```python
from build123d import *

# Parameters (mm, degrees)
F1_DEPTH = 6.35
F3_D     = 1.524
F4_R     = 0.381


with BuildPart() as f1:
    # F0 (on Front) → F1 (new body)
    with BuildSketch(Plane.XZ):
        with BuildLine():
            Line((0, -7.4092204591), (0, 0))
            Line((0, 0), (-2.54, 0))
            Line((-2.54, 0), (-2.54, -4.318))
            ThreePointArc((-2.54, -4.318), (-2.9863692655, -5.3956307345), (-4.064, -5.842))
            Line((-4.064, -5.842), (-9.398, -5.842))
            Line((-9.398, -5.842), (-11.068511021, -7.3997767286))
            ThreePointArc((-11.068511021, -7.3997767286), (-5.53701683, -10.6408992323), (0, -7.4092204591))
        make_face()
    extrude(amount=F1_DEPTH)

    # F3 (through all)
    with Locations(Plane.YZ):
        with Locations((-3.175, -1.7639952663)):
            Hole(F3_D / 2)

    # F4
    f4_edges = [f1.edges().sort_by_distance(p)[0] for p in [
        (-2.54, -3.175, 0),
        (0, -3.175, 0),
        (-1.27, -6.35, 0),
        (-1.27, 0, 0),
        (0, -6.35, -3.70461),
        (-2.54, -6.35, -2.159),
        (-2.986369, -6.35, -5.395631),
        (-6.731, -6.35, -5.842),
        (-10.233256, -6.35, -6.620888),
        (-5.537017, -6.35, -10.640899),
        (0, -3.175, -7.40922),
        (-9.398, -3.175, -5.842),
        (-2.54, 0, -2.159),
        (-2.986369, 0, -5.395631),
        (-6.731, 0, -5.842),
        (-10.233256, 0, -6.620888),
        (-5.537017, 0, -10.640899),
        (0, 0, -3.70461),
        (-11.068511, -3.175, -7.399777),
        (0, -3.937, -1.763995),
        (-2.54, -3.937, -1.763995),
    ]]
    fillet(f4_edges, radius=F4_R)


solid = f1.part
```
Design review of the part built by this model. Coordinates are the model's own, in mm. A direction names the side the tool comes from. Round coordinates to 2 decimals unless told otherwise and drop trailing zeros. Order: outer loops, then holes, each group sorted by start corner. A loop starts at its lowest first (then second) coordinate and runs counter-clockwise, first axis right, second up. Notation, with made-up numbers: (-19.5, 21) - (29.5, 21) arc R10 cw to (29.5, 39) - close; hole circle Ø9 at (33.5, 27). An arc over 180 degrees is marked (long way). One line per question, with ' | ' between items.
Item 1: Draft analysis for pull direction Y (two halves, no side actions). For faces 3 (the face through (-10.11, -6.24, -6.66)), 4 (the face through (-1.28, -3.58, -1.12)), 5 (the face through (-10.11, -0.11, -6.66)), 6 (the face through (-5.52, -3.14, -10.64)), state which applies: +Y half, -Y half, draft (parallel to the pull), parting line (faces both ways), or undercut.
Checks:
face 3: -Y half | face 4: undercut | face 5: +Y half | face 6: draft
Item 2: For P1, Ø2, axis at y = -4, z = -3, coming from the -X side, flat-tipped, find the tip position at first contact; note if it passes through.
Checks:
P1: x = -2.54
Item 3: Wall thickness on line 1 (X direction, y = -1, z = -0.75); line 2 (X direction, y = -3.5, z = -7.5); line 3 (Z direction, x = -2, y = -2.5): over which ranges is each line inside the solid? List them lowest first. Write a range as [from, to].
Checks:
line 1: [-2.54, 0] | line 2: [-10.96, -0.05] | line 3: [-9.57, -2.12], [-1.41, 0]
Item 4: Machinability: for faces 1 (the face through (-4, 0, -7)), 2 (the face through (-7, -3, -5.842)), which of the approach directions +Z, -Z, +X, -X, +Y, -Y give a long, thin tool a straight path to every point of the face, cutting with its end or side? Answer none if there is none.
Checks:
face 1: +Z, -Z, +X, -X, +Y | face 2: +Z, -X, +Y, -Y
Item 5: Take a section at A-A, the plane y = -1.5. Write out the cut boundary in (x, z).
Checks:
outline: (-10.91, -7.67) arc R6.35 ccw to (-0.05, -7.5) arc R0.38 ccw to (0, -7.31) - (0, -0.38) arc R0.38 ccw to (-0.38, 0) - (-2.16, 0) arc R0.38 ccw to (-2.54, -0.38) - (-2.54, -4.32) arc R1.52 cw to (-4.06, -5.84) - (-9.25, -5.84) arc R0.38 ccw to (-9.51, -5.94) - (-10.84, -7.19) arc R0.38 ccw to start
